Source: CAD feature listing. Evaluate the final solid. Frame: model axes, mm. Coordinates: 2 decimals unless noted, no trailing zeros. Order: outer loops, then holes, each group sorted by start corner. A loop starts at its lowest first (then second) coordinate and runs counter-clockwise, first axis right, second up.
```python
from build123d import *

# Parameters (mm, degrees)
SKETCH_R      = 2.54
EXTRUDE_DEPTH = 3.175


with BuildPart() as part:
    # Sketch → Extrude (new body)
    with BuildSketch(Plane.XZ):
        with BuildLine():
            ThreePointArc((107.810934, -12.593804), (117.43413, -5.869789), (117.434117, 5.869815))
            Line((64.34813, 107.723789), (117.434117, 5.869815))
            ThreePointArc((64.34813, 107.723789), (53.086, 114.554), (41.82387, 107.723789))
            Line((-11.26213, 5.869789), (41.82387, 107.723789))
            ThreePointArc((-11.26213, 5.869789), (-11.26213, -5.869789), (-1.638963, -12.5938))
            Line((-1.638963, -12.5938), (107.810934, -12.593804))
        make_face()
        with Locations((53.086, 33.951333)):
            Circle(SKETCH_R, mode=Mode.SUBTRACT)
    extrude(amount=EXTRUDE_DEPTH)


solid = part.part
```
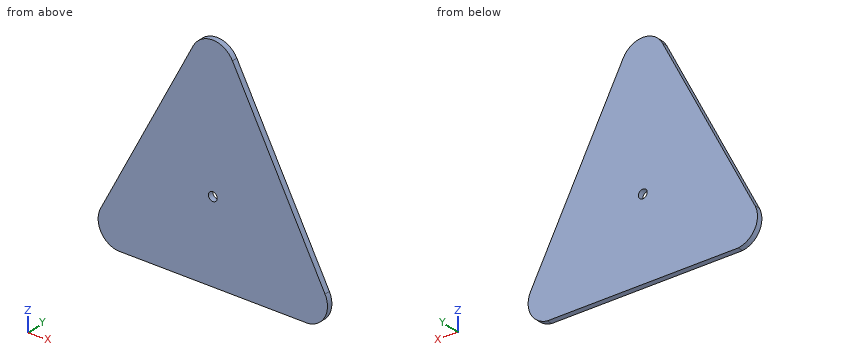
Q1. Material intervals for line 1 along X through (y, z) = (-1.75, 47); line 2 along Z through (x, y) = (59.5, -0.55); line 3 along Z through (x, y) = (4, -1.35), sorted ascending.
Solutions:
line 1: x = 10.17 to 96
line 2: z = -12.59 to 112.82
line 3: z = -12.59 to 35.15
Q2. Section query A-A on y = -0.75. Output: boundary loops of the cut face in (x, z).
Solutions:
outline: (-11.26, 5.87) arc R12.7 ccw to (-1.64, -12.59) - (107.81, -12.59) arc R12.7 ccw to (117.43, 5.87) - (64.35, 107.72) arc R12.7 ccw to (41.82, 107.72) - close; hole circle Ø5.08 at (53.09, 33.95)
Q3. Section query C-C on z = 65. Output: boundary loops of the cut face in (x, y) (3 decimals).
Solutions:
outline: (19.556, -3.175) - (86.616, -3.175) - (86.616, 0) - (19.556, 0) - close
Q4. Section query B-B on x = 100. Output: boundary loops of the cut face in (y, z) (3 decimals), plus the area to 3 significant figures.
Solutions:
outline: (-3.175, -12.594) - (0, -12.594) - (0, 39.32) - (-3.175, 39.32) - close
area: 165 mm2
